CAD build for the part. Positions are in the model's coordinates, mm. Round coordinates to 2 decimals unless told otherwise and drop trailing zeros. Order: outer loops, then holes, each group sorted by start corner. A loop starts at its lowest first (then second) coordinate and runs counter-clockwise, first axis right, second up. Notation, with made-up numbers: M 14.25,-6 L 64.25,-6 A19 cw 64.25,9 Z; hole C -16.75,88 d9. An arc over 180 degrees is marked long. Answer as a JSON object with one key per item and string values. Group by question number.
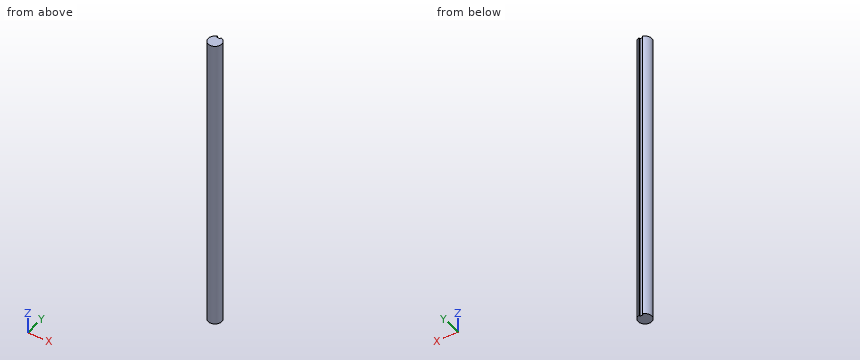
Autodesk Inventor part; units mm, degrees
ref_plane "YZ Plane" through (0, 0, 0) normal (1, 0, 0) x (0, 1, 0)
ref_plane "XZ Plane" through (0, 0, 0) normal (0, 1, 0) x (-1, 0, 0)
ref_plane "XY Plane" through (0, 0, 0) normal (0, 0, 1) x (1, 0, 0)
sketch "Sketch1" plane through (0, 0, 0) normal (0, 0, 1) x (1, 0, 0)
  circle A0 centre (0, 0) radius 6.35
  line L0 (-1.5875, 7.9375) -> (1.5875, 7.9375)
  line L1 (1.5875, 7.9375) -> (1.5875, 4.7625)
  line L2 (1.5875, 4.7625) -> (-1.5875, 4.7625)
  line L3 (-1.5875, 4.7625) -> (-1.5875, 7.9375)
  line L4 (1.5875, 4.7625) -> (1.5875, 6.1484)
  line L5 (-1.5875, 4.7625) -> (-1.5875, 6.1484)
  line L6 (1.5875, 4.7625) -> (-1.5875, 4.7625)
  point P0 (0, 4.7625)
  dimension "d0" = 12.7
  dimension "d1" = 3.175
  dimension "d2" = 3.175
  dimension "d3" = 4.7625
extrude "Extrusion1" add sketch "Sketch1" against normal blind 279.4 contours A0 L3 L2 L1 picked at (0.1781, 1.0658)
properties part number "11in axle"
Item 1: Drill centre lines: line 1 (X direction, y = 5.5, z = -178.5); line 2 (Y direction, x = 0.75, z = -108); line 3 (X direction, y = -0.25, z = -64.5). Where is each one in solid material? Low to high. Write a range as [from, to].
Item 2: Flat gauge pins, fed straight in: pin 1 Ø2 at (x, z) = (4.5, -83.5) entering from -Y; pin 2 Ø0.7 at (y, z) = (5.5, -208.5) entering from -X; pin 3 Ø3 at (x, z) = (-4, -140) entering from +Y. Where does each tip first touch, or does it go through?
Item 3: Cut at A-A, the plane x = -3.5. Give the cut face in (y, z).
Item 4: Cut at B-B, the plane y = -2.5. Give the cut face in (x, z), and give its area (3 significant figures).
Response values:
{
 "1": {"line 1": "[-3.17, -1.59], [1.59, 3.17]", "line 2": "[-6.31, 4.76]", "line 3": "[-6.35, 6.35]"},
 "2": {"pin 1": "y = -5.3", "pin 2": "x = -3.71", "pin 3": "y = 5.84"},
 "3": {"outline": "M -5.3,-279.4 L 5.3,-279.4 L 5.3,0 L -5.3,0 Z"},
 "4": {"outline": "M -5.84,-279.4 L 5.84,-279.4 L 5.84,0 L -5.84,0 Z", "area": "3,260 mm^2"}
}
